Can you work these out from the model? Positions are in its coordinate system, mm. Give positions to 0.01 mm unless a question says otherwise; leave off trailing zeros. Order: outer loops, then holes, each group sorted by start corner. A loop starts at its lowest first (then second) coordinate and runs counter-clockwise, first axis right, second up. Notation, with made-up numbers: (32.25, 33) - (72.25, 33) arc R16 ccw to (72.25, 48) - close; hole circle Ø3 at (-20, -6). An arc over 180 degrees is marked (long way). One line per question, with ' | ' between items.
```python
from build123d import *

# Parameters (mm, degrees)
F0_W     = 2082.8
F0_H     = 914.4
F2_DEPTH = 9.525
F1_W     = 699.5541
F1_H     = 904.875
F1_W_2   = 626.5418
F3_DEPTH = 9.525


with BuildPart() as f2:
    # F0 (on Top) → F2 (new body)
    with BuildSketch(Plane.XY):
        Rectangle(F0_W, F0_H)
    extrude(amount=F2_DEPTH)

    # F1 (on Top) → F3 (join)
    with BuildSketch(Plane.XY):
        with Locations((-682.09795, -4.7625)):
            Rectangle(F1_W, F1_H)
        with Locations((682.09795, -4.7625)):
            Rectangle(F1_W, F1_H)
        with Locations((0, -4.7625)):
            Rectangle(F1_W_2, F1_H)
    extrude(amount=-F3_DEPTH)


solid = f2.part
```
(1) If I drill on line 1 (X direction, y = 291, z = -8.5) (3 decimals); line 2 (Y direction, x = -613.5, z = -8.25) (3 decimals), over which ranges is the centre line in solid material (lowest first)?
Answer below:
line 1: -1031.875 to -332.321, -313.271 to 313.271, 332.321 to 1031.875 | line 2: -457.2 to 447.675
(2) Will these pins go through, and if not, where does the flat tip stop? pin 1 (3 mm diameter, centred on x = 594, z = -5.5, fed in from +Y) (3 decimals); pin 2 (2 mm diameter, centred on y = 183.5, z = -7.5, fed in from -X) (3 decimals); pin 3 (3 mm diameter, centred on y = 109.5, z = -6.5, fed in from +X) (3 decimals).
Answer below:
pin 1: y = 447.675 | pin 2: x = -1031.875 | pin 3: x = 1031.875
(3) If we mould it in two halves opening along X, with no side actions, what happens to faces 1 (the face through (-687, 2, -9.525)), 2 (the face through (-313.423, 2.134, 0))? For each: released by +X, released by -X, zero draft, split by the parting line, or undercut.
Answer below:
face 1: zero draft | face 2: undercut
(4) Imagine slicing it at A-A (z = -6). List the corners of the cut face in (x, y) for me (3 decimals), and give its area (3 significant figures).
Answer below:
outline: (-1031.875, -457.2) - (-332.321, -457.2) - (-332.321, 447.675) - (-1031.875, 447.675) - close; (-313.271, -457.2) - (313.271, -457.2) - (313.271, 447.675) - (-313.271, 447.675) - close; (332.321, -457.2) - (1031.875, -457.2) - (1031.875, 447.675) - (332.321, 447.675) - close | area: 1,830,000 mm^2
